The listing builds one solid part. Answer for the finished solid, in the listing's coordinates (mm). A direction names the side the tool comes from. Coordinates: 2 decimals unless noted, no trailing zeros. Order: outer loops, then holes, each group sorted by start corner. A loop starts at its lowest first (then second) coordinate and runs counter-clockwise, first axis right, second up. Notation, with made-up numbers: (74.25, 14.5) - (112.25, 14.5) arc R21 ccw to (112.25, 40.5) - close; hole circle Ø7 at (15, -15). An arc over 180 degrees is marked (long way). Use one line per item in the form item = value. Start each with the question number.
Item 1: Section C-C, the plane y = 13 is taken. Write down the section's boundary in (x, z).
Item 2: Consider line 1 along Y through (x, z) = (-20.5, -0.7) (3 decimals); line 2 along Y through (x, z) = (-78.5, -1.6) (3 decimals); line 3 along Y through (x, z) = (-4, 10). Determine where each line is inside the solid, lowest interval first. Write a range as [from, to].
Item 3: Section A-A, the plane z = 10.75 is taken. Write down the section's boundary in (x, y).
Item 4: Each of these flat-tipped pins is pushed along its axis until it touches: pin 1 Ø8 at (x, z) = (-58, 4) entering from -Y; pin 2 Ø4.5 at (x, z) = (-5, 12.5) entering from +Y; pin 3 Ø12 at (x, y) = (-70.5, 19.5) entering from +Z. Where does it stop, or does it pass through?
Item 5: The mould has two halves that part along X. Classify faces 4 (the flat face through (-3, 19.75, 9)), 5 (the cylindrical face through (-81.14, -2.1, -0.4)), 6 (the flat face through (-67.7, -2, 3)): released by +X, released by -X, zero draft, split by the parting line, or undercut.
Item 6: A tool of negligible diameter and unlimited length cuts with its end or side. For faces 1 (the flat face through (-50, 7.1, 5)), 2 (the cylindrical face through (2.14, 52.1, -0.4)), 3 (the flat face through (-77, 26, -1.4)), from which of +Z, -Z, +X, -X, +Y, -Y can it reach the whole face along a straight path? Write none if from no direction.
Item 7: Section D-D, the plane x = -59 is taken. Write down the section's boundary in (y, z).
Item 8: Section B-B, the plane x = -20.5 is taken. Write down the section's boundary in (y, z) (3 decimals), and give its area (3 significant figures).
Autodesk Fusion 360 part; units mm, degrees
sketch "Sketch1" plane through (0, 0, 0) normal (0, 0, 1) x (1, 0, 0)
  line L0 (0, -3) -> (-79, -3)
  line L1 (-82, 0) -> (-82, 50)
  line L2 (-79, 53) -> (0, 53)
  line L3 (3, 50) -> (3, 0)
  arc A0 (-79, 53) -> (-82, 50) centre (-79, 50) ccw
  arc A1 (-82, 0) -> (-79, -3) centre (-79, 0) ccw
  arc A2 (3, 50) -> (0, 53) centre (0, 50) ccw
  arc A3 (0, -3) -> (3, 0) centre (0, 0) ccw
  circle A4 centre (-78.5, 49.5) radius 1.375
  circle A5 centre (-78.5, 0.5) radius 1.375
  circle A6 centre (-20.5, 49.5) radius 1.375
  circle A7 centre (-20.5, 0.5) radius 1.375
  dimension "d1" = 3
  dimension "d2" = 85
  dimension "d3" = 56
  dimension "d4" = 49
  dimension "d5" = 0.5
  dimension "d6" = 0.5
  dimension "d7" = 2.75
  dimension "d8" = 2.75
  dimension "d9" = 3.5
  dimension "d10" = 2.75
  dimension "d11" = 2.75
  dimension "d12" = 58
  dimension "d13" = 58
  dimension "d14" = 49
  dimension "d15" = 49
extrude "Extrude1" add sketch "Sketch1" along normal blind 1.6
sketch "Sketch2" plane through (0, 0, 0) normal (0, 0, -1) x (1, 0, 0)
  circle A0 centre (-20.5, -49.5) radius 1.375
  circle A1 centre (-78.5, -0.5) radius 1.375
  circle A2 centre (-20.5, -0.5) radius 1.375
  circle A3 centre (-78.5, -49.5) radius 1.375
  arc A4 (-79, 3) -> (-82, 0) centre (-79, 0) ccw
  line L0 (-82, 0) -> (-82, -50)
  arc A5 (-82, -50) -> (-79, -53) centre (-79, -50) ccw
  line L1 (-79, -53) -> (0, -53)
  arc A6 (0, -53) -> (3, -50) centre (0, -50) ccw
  line L2 (3, -50) -> (3, 0)
  arc A7 (3, 0) -> (0, 3) centre (0, 0) ccw
  line L3 (0, 3) -> (-79, 3)
  line L4 (-67.4, -18.5) -> (-85.4, -18.5)
  line L5 (-85.4, -18.5) -> (-85.4, -33.1)
  line L6 (-85.4, -33.1) -> (-67.4, -33.1)
  line L7 (-67.4, -33.1) -> (-67.4, -18.5)
  dimension "d18" = 14.6
  dimension "d19" = 19.9
  dimension "d20" = 18
  dimension "d21" = 3.4
extrude "Extrude2" add sketch "Sketch2" along normal blind 1.4 contours L0 L4 L6 L7 | L0 L4 L5 L6
extrude "Extrude3" add 1 faces at (-36.7049, 22.8333, 0) along direction (0, 0, -1) blind 2.45
sketch "Sketch3" plane through (0, 0, 1.6) normal (0, 0, 1) x (-1, 0, 0)
  circle A0 centre (20.5, -49.5) radius 1.375
  circle A1 centre (78.5, -0.5) radius 1.375
  circle A2 centre (20.5, -0.5) radius 1.375
  circle A3 centre (78.5, -49.5) radius 1.375
  arc A4 (82, 0) -> (79, 3) centre (79, 0) ccw
  line L0 (79, 3) -> (0, 3)
  arc A5 (0, 3) -> (-3, 0) centre (0, 0) ccw
  line L1 (-3, 0) -> (-3, -50)
  arc A6 (-3, -50) -> (0, -53) centre (0, -50) ccw
  line L2 (0, -53) -> (79, -53)
  arc A7 (79, -53) -> (82, -50) centre (79, -50) ccw
  line L3 (82, -50) -> (82, 0)
  line L4 (31.5, -9.5) -> (25.5, -9.5)
  line L5 (25.5, -9.5) -> (25.5, 3)
  line L6 (25.5, 3) -> (31.5, 3)
  line L7 (31.5, 3) -> (31.5, -9.5)
  line L8 (57.5, -7.1) -> (42.5, -7.1)
  line L9 (42.5, -7.1) -> (42.5, 4.5)
  line L10 (42.5, 4.5) -> (57.5, 4.5)
  line L11 (57.5, 4.5) -> (57.5, -7.1)
  line L12 (75.2, -1.2) -> (67.7, -1.2)
  line L13 (67.7, -1.2) -> (67.7, 4.5)
  line L14 (67.7, 4.5) -> (75.2, 4.5)
  line L15 (75.2, 4.5) -> (75.2, -1.2)
  dimension "d26" = 7.5
  dimension "d27" = 10.2
  dimension "d28" = 15
  dimension "d29" = 11
  dimension "d30" = 6
  dimension "d31" = 28.5
  dimension "d32" = 12.5
  dimension "d33" = 1.5
  dimension "d34" = 1.5
  dimension "d35" = 11.6
  dimension "d36" = 5.7
extrude "Extrude4" add sketch "Sketch3" along normal blind 6.5 contours L0 L8 L9 L11 | L0 L9 L10 L11 | L0 L4 L5 L6 L7
extrude "Extrude5" add sketch "Sketch3" along normal blind 2.45 contours L0 L12 L13 L15 | L0 L13 L14 L15
sketch "Sketch4" plane through (0, -3, 0) normal (0, -1, 0) x (1, 0, 0)
  line L0 (0, -2.45) -> (0, 1.6)
  line L1 (0, 1.6) -> (-25.5, 1.6)
  line L2 (-25.5, 1.6) -> (-25.5, 8.1)
  line L3 (-25.5, 8.1) -> (-31.5, 8.1)
  line L4 (-31.5, 8.1) -> (-31.5, 1.6)
  line L5 (-31.5, 1.6) -> (-42.5, 1.6)
  line L6 (-42.5, 1.6) -> (-57.5, 1.6)
  line L7 (-57.5, 1.6) -> (-67.7, 1.6)
  line L8 (-67.7, 1.6) -> (-75.2, 1.6)
  line L9 (-75.2, 1.6) -> (-79, 1.6)
  line L10 (-79, 1.6) -> (-79, -2.45)
  line L11 (-79, -2.45) -> (0, -2.45)
  circle A0 centre (-28.5, 4.64) radius 3
  line L12 (-25.5, 1.6) -> (-31.5, 1.6)
  dimension "d41" = 6
  dimension "d42" = 3
  dimension "d43" = 3.04
extrude "Extrude6" add sketch "Sketch4" along normal blind 2.5 contours A0
sketch "Sketch5" plane through (0, 0, 1.6) normal (0, 0, 1) x (1, 0, 0)
  line L0 (5.1, -0.25) -> (-16.3, -0.25)
  line L1 (-16.3, -0.25) -> (-16.3, 15.75)
  line L2 (-16.3, 15.75) -> (5.1, 15.75)
  line L3 (5.1, 15.75) -> (5.1, -0.25)
  line L4 (5.1, 19.75) -> (-12.1, 19.75)
  line L5 (-12.1, 19.75) -> (-12.1, 33.05)
  line L6 (-12.1, 33.05) -> (5.1, 33.05)
  line L7 (5.1, 33.05) -> (5.1, 19.75)
  line L8 (5.1, 37.55) -> (-12.1, 37.55)
  line L9 (-12.1, 37.55) -> (-12.1, 50.85)
  line L10 (-12.1, 50.85) -> (5.1, 50.85)
  line L11 (5.1, 50.85) -> (5.1, 37.55)
  line L12 (3, 0) -> (3, 50)
  line L13 (-79, -3) -> (0, -3)
  dimension "d46" = 13.3
  dimension "d47" = 13.3
  dimension "d48" = 16
  dimension "d49" = 2.1
  dimension "d50" = 2.1
  dimension "d51" = 2.1
  dimension "d52" = 4.5
  dimension "d53" = 4
  dimension "d54" = 2.75
  dimension "d55" = 21.4
  dimension "d56" = 17.2
  dimension "d57" = 17.2
extrude "Extrude7" add sketch "Sketch5" along normal blind 15.5 contours L8 L9 L10 L11 | L4 L5 L6 L12 | L4 L6 L7 L12
extrude "Extrude8" add sketch "Sketch5" along normal blind 13.8 contours L0 L1 L2 L3
sketch "Sketch6" plane through (0, 0, 1.6) normal (0, 0, 1) x (-1, 0, 0)
  line L0 (16.3, -15.75) -> (-3, -15.75)
  line L1 (-3, -15.75) -> (-3, -19.75)
  line L2 (-3, -19.75) -> (12.1, -19.75)
  line L3 (12.1, -19.75) -> (12.1, -33.05)
  line L4 (12.1, -33.05) -> (-3, -33.05)
  line L5 (-3, -33.05) -> (-3, -37.55)
  line L6 (-3, -37.55) -> (12.1, -37.55)
  line L7 (12.1, -37.55) -> (12.1, -50.85)
  line L8 (12.1, -50.85) -> (-2.8771, -50.85)
  arc A0 (-2.8771, -50.85) -> (0, -53) centre (0, -50) ccw
  line L9 (0, -53) -> (79, -53)
  arc A1 (79, -53) -> (82, -50) centre (79, -50) ccw
  line L10 (82, -50) -> (82, 0)
  arc A2 (82, 0) -> (79, 3) centre (79, 0) ccw
  line L11 (79, 3) -> (75.2, 3)
  line L12 (75.2, 3) -> (75.2, -1.2)
  line L13 (75.2, -1.2) -> (67.7, -1.2)
  line L14 (67.7, -1.2) -> (67.7, 3)
  line L15 (67.7, 3) -> (57.5, 3)
  line L16 (57.5, 3) -> (57.5, -7.1)
  line L17 (57.5, -7.1) -> (42.5, -7.1)
  line L18 (42.5, -7.1) -> (42.5, 3)
  line L19 (42.5, 3) -> (31.5, 3)
  line L20 (31.5, 3) -> (31.5, -9.5)
  line L21 (31.5, -9.5) -> (25.5, -9.5)
  line L22 (25.5, -9.5) -> (25.5, 3)
  line L23 (25.5, 3) -> (0, 3)
  arc A3 (0, 3) -> (-2.9896, 0.25) centre (0, 0) ccw
  line L24 (-2.9896, 0.25) -> (16.3, 0.25)
  line L25 (16.3, 0.25) -> (16.3, -15.75)
  circle A4 centre (20.5, -49.5) radius 1.375
  circle A5 centre (78.5, -0.5) radius 1.375
  circle A6 centre (20.5, -0.5) radius 1.375
  circle A7 centre (78.5, -49.5) radius 1.375
  line L26 (75.2, -51.94) -> (24.2, -51.94)
  line L27 (24.2, -51.94) -> (24.2, -46.94)
  line L28 (24.2, -46.94) -> (75.2, -46.94)
  line L29 (75.2, -46.94) -> (75.2, -51.94)
  dimension "d62" = 6.8
  dimension "d63" = 1.06
  dimension "d64" = 51
  dimension "d65" = 5
extrude "Extrude9" add sketch "Sketch6" along normal blind 8.1 contours L26 L27 L28 L29
sketch "Sketch7" plane through (0, 0, 1.6) normal (0, 0, 1) x (-1, 0, 0)
  line L0 (75.2, -46.94) -> (75.2, -51.94)
  line L1 (75.2, -51.94) -> (24.2, -51.94)
  line L2 (24.2, -51.94) -> (24.2, -46.94)
  line L3 (24.2, -46.94) -> (75.2, -46.94)
  line L4 (16.3, -15.75) -> (-3, -15.75)
  line L5 (-3, -15.75) -> (-3, -19.75)
  line L6 (-3, -19.75) -> (12.1, -19.75)
  line L7 (12.1, -19.75) -> (12.1, -33.05)
  line L8 (12.1, -33.05) -> (-3, -33.05)
  line L9 (-3, -33.05) -> (-3, -37.55)
  line L10 (-3, -37.55) -> (12.1, -37.55)
  line L11 (12.1, -37.55) -> (12.1, -50.85)
  line L12 (12.1, -50.85) -> (-2.8771, -50.85)
  arc A0 (-2.8771, -50.85) -> (0, -53) centre (0, -50) ccw
  line L13 (0, -53) -> (79, -53)
  arc A1 (79, -53) -> (82, -50) centre (79, -50) ccw
  line L14 (82, -50) -> (82, 0)
  arc A2 (82, 0) -> (79, 3) centre (79, 0) ccw
  line L15 (79, 3) -> (75.2, 3)
  line L16 (75.2, 3) -> (75.2, -1.2)
  line L17 (75.2, -1.2) -> (67.7, -1.2)
  line L18 (67.7, -1.2) -> (67.7, 3)
  line L19 (67.7, 3) -> (57.5, 3)
  line L20 (57.5, 3) -> (57.5, -7.1)
  line L21 (57.5, -7.1) -> (42.5, -7.1)
  line L22 (42.5, -7.1) -> (42.5, 3)
  line L23 (42.5, 3) -> (31.5, 3)
  line L24 (31.5, 3) -> (31.5, -9.5)
  line L25 (31.5, -9.5) -> (25.5, -9.5)
  line L26 (25.5, -9.5) -> (25.5, 3)
  line L27 (25.5, 3) -> (0, 3)
  arc A3 (0, 3) -> (-2.9896, 0.25) centre (0, 0) ccw
  line L28 (-2.9896, 0.25) -> (16.3, 0.25)
  line L29 (16.3, 0.25) -> (16.3, -15.75)
  circle A4 centre (20.5, -49.5) radius 1.375
  circle A5 centre (78.5, -0.5) radius 1.375
  circle A6 centre (20.5, -0.5) radius 1.375
  circle A7 centre (78.5, -49.5) radius 1.375
  line L30 (62, -35.5) -> (48, -35.5)
  line L31 (48, -35.5) -> (48, -21.5)
  line L32 (48, -21.5) -> (62, -21.5)
  line L33 (62, -21.5) -> (62, -35.5)
  line L34 (79, -53) -> (0, -53)
  line L35 (82, 0) -> (82, -50)
  dimension "d68" = 31.5
  dimension "d69" = 34
  dimension "d70" = 14
  dimension "d71" = 14
extrude "Extrude10" add sketch "Sketch7" along normal blind 1 contours L30 L31 L32 L33
equation "d8 = d7"
equation "d10 = d7"
equation "d11 = d7"
equation "d13 = d12"
equation "d14 = d4"
equation "d15 = d4"
equation "d21 = d20 - 14.6 mm"
equation "d47 = d46"
equation "d50 = d49"
equation "d51 = d49"
equation "d57 = d56"
Response:
q1.outline = (-82, -2.45) - (3, -2.45) - (3, 1.6) - (5.1, 1.6) - (5.1, 15.4) - (-16.3, 15.4) - (-16.3, 1.6) - (-82, 1.6) - close
q2.line_1 = [-3, -0.875], [1.875, 48.125], [50.875, 53]
q2.line_2 = [-3, -0.875], [1.875, 18.5], [33.1, 48.125], [50.875, 53]
q2.line_3 = [-0.25, 15.75], [19.75, 33.05], [37.55, 50.85]
q3.outline = (-16.3, -0.25) - (5.1, -0.25) - (5.1, 15.75) - (-16.3, 15.75) - close; (-12.1, 19.75) - (5.1, 19.75) - (5.1, 33.05) - (-12.1, 33.05) - close; (-12.1, 37.55) - (5.1, 37.55) - (5.1, 50.85) - (-12.1, 50.85) - close
q4.pin_1 = -4.5
q4.pin_2 = 50.85
q4.pin_3 = 1.6
q5.face_4 = zero draft
q5.face_5 = released by -X
q5.face_6 = undercut
q6.face_1 = +Z, -X
q6.face_2 = -Z, +X, +Y
q6.face_3 = -Z, -X
q7.outline = (-3, -2.45) - (53, -2.45) - (53, 1.6) - (51.94, 1.6) - (51.94, 9.7) - (46.94, 9.7) - (46.94, 1.6) - (35.5, 1.6) - (35.5, 2.6) - (21.5, 2.6) - (21.5, 1.6) - (-3, 1.6) - close
q8.outline = (-3, -2.45) - (-0.875, -2.45) - (-0.875, 1.6) - (-3, 1.6) - close; (1.875, -2.45) - (48.125, -2.45) - (48.125, 1.6) - (1.875, 1.6) - close; (50.875, -2.45) - (53, -2.45) - (53, 1.6) - (50.875, 1.6) - close
q8.area = 205 mm2
